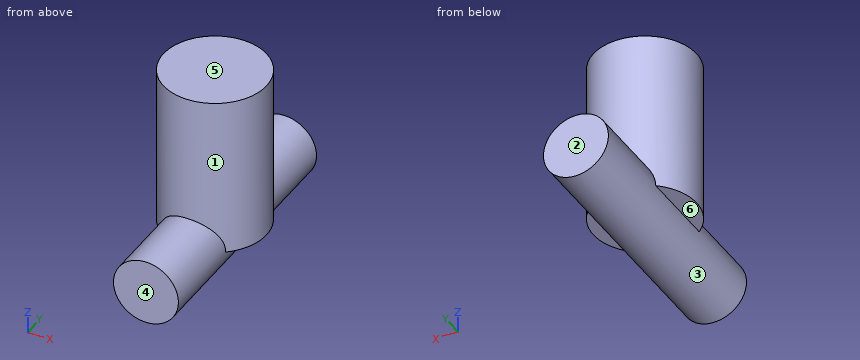
from build123d import *

# Parameters (mm, degrees)
BOSS_EXTRUDE1_DEPTH      = 31.35
BOSS_EXTRUDE1_DEPTH_BACK = 31.35
SKETCH1_R                = 8
SKETCH2_R                = 12.7
BOSS_EXTRUDE2_DEPTH      = 39.5


with BuildPart() as part:
    # Sketch1 → Boss-Extrude1 (new, two sides: drawn at the far end of the back side and taken through both)
    with BuildSketch(Plane(origin=(0, 0, 0), x_dir=(1, 0, 0), z_dir=(0, 1, 0)).offset(-BOSS_EXTRUDE1_DEPTH_BACK)):
        with Locations(Location((0, 0, 0), (0, 0, 270))):
            Circle(SKETCH1_R)
    extrude(amount=BOSS_EXTRUDE1_DEPTH + BOSS_EXTRUDE1_DEPTH_BACK)

    # Sketch2 → Boss-Extrude2 (add)
    with BuildSketch(Plane.XY):
        with Locations(Location((0, 0, 0), (0, 0, 129.044313469))):
            Circle(SKETCH2_R)
    extrude(amount=BOSS_EXTRUDE2_DEPTH)


solid = part.part
Verification items for the finished model (mm, model axes). Face numbers are marked on the shaded views. A direction names the side the tool comes from. Coordinates: 2 decimals unless noted, no trailing zeros. Order: outer loops, then holes, each group sorted by start corner. A loop starts at its lowest first (then second) coordinate and runs counter-clockwise, first axis right, second up. Notation, with made-up numbers: M 52.25,-3.5 L 67.25,-3.5 A33 cw 67.25,31.5 Z; hole C -6,62 d9. An arc over 180 degrees is marked long. One line per item, written item: value. Start each with the question number.
Item 1: Thickness scan on probe 1 along Z at (x, y) = (10.75, 4); probe 2 along X at (y, z) = (8, 15); probe 3 along Z at (x, y) = (-6.75, 14.5). Record the ranges inside material, lowest first.
Item 2: Sectioned sample at B-B on y = 0. Record the cut outline in (x, z).
Item 3: Sectioned sample at D-D on x = 4. Record the cut outline in (y, z).
Item 4: Sectioned sample at C-C on z = 17. Record the cut outline in (x, y).
Item 5: Depth check by flat-ended pin: P1, Ø5, axis at x = -9.5, y = 4.5, coming from the -Z side; P2, Ø6, axis at y = 0.5, z = 0.5, coming from the +X side; P3, Ø3, axis at x = 6, y = -1, coming from the -Z side; P4, Ø12, axis at y = -19.5, z = 13, coming from the +X side. Enter the tip coordinate at first touch or a pass-through.
Item 6: Mould release check, pull along Z, two halves, no side actions. Record for the marked faces 3, 4, 5 and 6: pulls with the +Z half, pulls with the -Z half, needs draft (parallel to the pull), parting line crosses it, or undercut.
Item 7: Access from +Z, -Z, +X, -X, +Y, -Y to the whole of each face (thin tool, end or side, straight path). Record for the marked faces 1 and 2.
Item 8: Sectioned sample at A-A on x = 0. Record the cut outline in (y, z), then the cut area to 3 significant figures.
Calculated:
1. probe 1: 0 to 39.5
1. probe 2: -9.86 to 9.86
1. probe 3: -4.29 to 4.29
2. outline: M -12.7,0 L -8,0 A8 ccw 8,0 L 12.7,0 L 12.7,39.5 L -12.7,39.5 Z
3. outline: M -31.35,-6.93 L 31.35,-6.93 L 31.35,6.93 L 12.05,6.93 L 12.05,39.5 L -12.05,39.5 L -12.05,6.93 L -31.35,6.93 Z
4. outline: C 0,0 d25.4
5. P1: z = -3.87
5. P2: x = 12.7
5. P3: z = -6.61
5. P4: x = 3.87
6. face 3: parting line crosses it
6. face 4: needs draft
6. face 5: pulls with the +Z half
6. face 6: pulls with the -Z half
7. face 1: +Z
7. face 2: +Z, -Z, +X, -X, +Y
8. outline: M -31.35,-8 L 31.35,-8 L 31.35,8 L 12.7,8 L 12.7,39.5 L -12.7,39.5 L -12.7,8 L -31.35,8 Z
8. area: 1,800 mm^2
